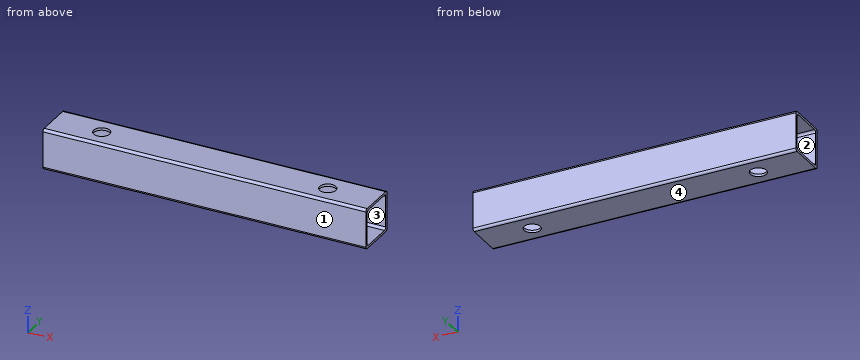
```python
from build123d import *

# Parameters (mm, degrees)
BOSS_EXTRUDE1_DEPTH = 200
SKETCH3_R           = 5
CUT_EXTRUDE1_DEPTH  = 204.100960116


with BuildPart() as part:
    # Sketch1 → Boss-Extrude1 (new body)
    with BuildSketch(Plane(origin=(0, 0, 0), x_dir=(0, 0, -1), z_dir=(1, 0, 0))):
        with BuildLine():
            Line((1.5, 0), (23.5, 0))
            ThreePointArc((23.5, 0), (24.560660172, 0.439339828), (25, 1.5))
            Line((25, 1.5), (25, 23.5))
            ThreePointArc((25, 23.5), (24.560660172, 24.560660172), (23.5, 25))
            Line((23.5, 25), (1.5, 25))
            ThreePointArc((1.5, 25), (0.439339828, 24.560660172), (0, 23.5))
            Line((0, 23.5), (0, 1.5))
            ThreePointArc((0, 1.5), (0.439339828, 0.439339828), (1.5, 0))
        make_face()
        with BuildLine():
            Line((3, 23.5), (22, 23.5))
            ThreePointArc((22, 23.5), (23.060660172, 23.060660172), (23.5, 22))
            Line((23.5, 22), (23.5, 3))
            ThreePointArc((23.5, 3), (23.060660172, 1.939339828), (22, 1.5))
            Line((22, 1.5), (3, 1.5))
            ThreePointArc((3, 1.5), (1.939339828, 1.939339828), (1.5, 3))
            Line((1.5, 3), (1.5, 22))
            ThreePointArc((1.5, 22), (1.939339828, 23.060660172), (3, 23.5))
        make_face(mode=Mode.SUBTRACT)
    extrude(amount=BOSS_EXTRUDE1_DEPTH)

    # Sketch3 → Cut-Extrude1 (cut, through all)
    with BuildSketch(Plane(origin=(0, 0, -25), x_dir=(-1, 0, 0), z_dir=(0, 0, -1))):
        with Locations((-170, 12.176713796)):
            Circle(SKETCH3_R)
        with Locations((-30, 12.176713796)):
            Circle(SKETCH3_R)
    extrude(amount=-CUT_EXTRUDE1_DEPTH, mode=Mode.SUBTRACT)


solid = part.part
```
The model under review builds one solid part; all positions refer to its coordinate system, in mm. Face numbers are marked on the shaded views. Coordinates: 2 decimals unless noted, no trailing zeros. Order: outer loops, then holes, each group sorted by start corner. A loop starts at its lowest first (then second) coordinate and runs counter-clockwise, first axis right, second up. Notation, with made-up numbers: M 37,48 L 84,48 A29 cw 84,83 Z; hole C -28,50 d6. An arc over 180 degrees is marked long. One line per question, with ' | ' between items.
(1) Add section D-D, the plane x = 160. Write out the cut boundary in (y, z), then the cut area to 3 significant figures.
Geometry results:
outline: M 0,-23.5 A1.5 ccw 1.5,-25 L 23.5,-25 A1.5 ccw 25,-23.5 L 25,-1.5 A1.5 ccw 23.5,0 L 1.5,0 A1.5 ccw 0,-1.5 Z; hole M 1.5,-22 A1.5 ccw 3,-23.5 L 22,-23.5 A1.5 ccw 23.5,-22 L 23.5,-3 A1.5 ccw 22,-1.5 L 3,-1.5 A1.5 ccw 1.5,-3 Z | area: 141 mm²
(2) Add section A-A, the plane y = 19.5. Write out the cut boundary in (x, z), then the cut area to 3 significant figures.
Geometry results:
outline: M 0,-25 L 200,-25 L 200,-23.5 L 0,-23.5 Z; M 0,-1.5 L 200,-1.5 L 200,0 L 0,0 Z | area: 600 mm²
(3) Add section C-C, the plane z = -19.25. Write out the cut boundary in (x, y).
Geometry results:
outline: M 0,0 L 200,0 L 200,1.5 L 0,1.5 Z; M 0,23.5 L 200,23.5 L 200,25 L 0,25 Z
(4) For probe 1 along Y at (x, z) = (24.5, -20.5); probe 2 along Z at (x, y) = (154, 10.5); probe 3 along X at (y, z) = (14.25, -1.25), list the stretches that pass through material, from the lowest coordinate up. Write a range as from..to.
Geometry results:
probe 1: y = 0..1.5, 23.5..25 | probe 2: z = -25..-23.5, -1.5..0 | probe 3: x = 0..25.45, 34.55..165.45, 174.55..200
(5) Add section B-B, the plane x = 30. Write out the cut boundary in (y, z).
Geometry results:
outline: M 0,-23.5 A1.5 ccw 1.5,-25 L 7.18,-25 L 7.18,-23.5 L 3,-23.5 A1.5 cw 1.5,-22 L 1.5,-3 A1.5 cw 3,-1.5 L 7.18,-1.5 L 7.18,0 L 1.5,0 A1.5 ccw 0,-1.5 Z; M 17.18,-25 L 23.5,-25 A1.5 ccw 25,-23.5 L 25,-1.5 A1.5 ccw 23.5,0 L 17.18,0 L 17.18,-1.5 L 22,-1.5 A1.5 cw 23.5,-3 L 23.5,-22 A1.5 cw 22,-23.5 L 17.18,-23.5 Z
(6) The part is to be moulded in two halves that separate along Z. For the marked faces 1, 2, 3 and 4, say which applies: +Z half, -Z half, draft (parallel to the pull), parting line (faces both ways), or undercut.
Geometry results:
face 1: draft | face 2: undercut | face 3: undercut | face 4: -Z half
